Part model, mm, in its own coordinate system. Round coordinates to 2 decimals unless told otherwise and drop trailing zeros. Write each loop counter-clockwise with the first axis right and the second up, starting at its lowest first coordinate (ties: lowest second). Pieces come first, ordered by that corner, then holes. Notation, with made-up numbers: M 89.25,46 L 103.25,46 A16 cw 103.25,53 Z; hole C 3,33 d7. An arc over 180 degrees is marked long. One line per question, with ' | ' between items. Start each with the question number.
1) Saw through at A-A (z = 0). List the corners of the cut face in (x, y).
2) Saw through at B-B (y = 11.75). List the corners of the cut face in (x, z).
3) Saw through at C-C (x = 31.5). List the corners of the cut face in (y, z).
4) Wall check: probe 1 along Z at (x, y) = (18, 0); probe 2 along X at (y, z) = (12.5, 0.05); probe 3 along Y at (x, z) = (27, 0.15). Give the ranges that are in metal, low to high. Write a range as [from, to].
Autodesk Fusion 360 part; units mm, degrees
sketch "Sketch1" plane through (0, 0, 0) normal (1, 0, 0) x (0, 1, 0)
  circle A0 centre (0, 0) radius 1.3
  circle A1 centre (0, 0) radius 1.1476
  dimension "d1" = 2.6
  dimension "d2" = 2.2952
extrude "Extrude1" add sketch "Sketch1" along normal blind 20
equation "d2 = d1 - 0.012 in"

Autodesk Fusion 360 part; units mm, degrees
sketch "Sketch1" plane through (0, 0, 0) normal (1, 0, 0) x (0, 1, 0)
  circle A0 centre (0, 0) radius 1.3
  circle A1 centre (0, 0) radius 1.1476
  dimension "d1" = 2.6
  dimension "d2" = 2.2952
extrude "Extrude1" add sketch "Sketch1" along normal blind 7
equation "d2 = d1 - 0.012 in"

Autodesk Fusion 360 part; units mm, degrees
sketch "Sketch1" plane through (0, 0, 0) normal (1, 0, 0) x (0, 1, 0)
  circle A0 centre (0, 0) radius 1.3
  circle A1 centre (0, 0) radius 1.1476
  dimension "d1" = 2.6
  dimension "d2" = 2.2952
sketch "Sketch2" plane through (0, 0, 0) normal (0, 0, 1) x (1, 0, 0)
  line L0 (0, 0) -> (40.8, 0)
  line L1 (50.8, 10) -> (50.8, 25)
  arc A0 (40.8, 0) -> (50.8, 10) centre (40.8, 10) ccw
  point P0 (50.8, 0)
  dimension "d3" = 50.8
  dimension "d4" = 25
  dimension "d5" = 10
sweep "Sweep1" add profiles "Sketch1" path "Sketch2" along L0 A0 L1 section 1
equation "d2 = d1 - 0.012 in"
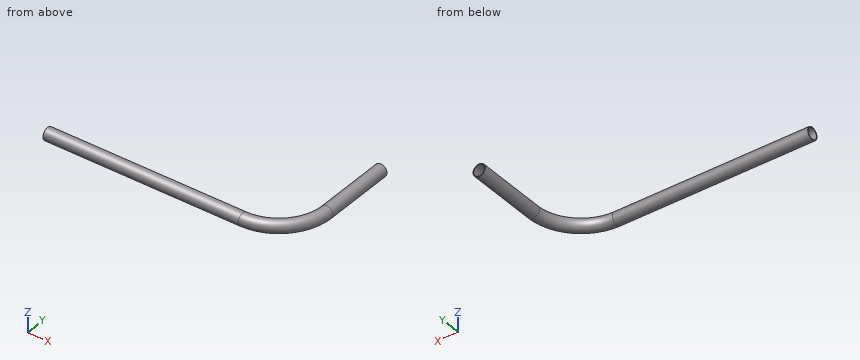
Answer key:
1) outline: M 0,-1.3 L 40.8,-1.3 A11.3 ccw 52.1,10 L 52.1,25 L 51.95,25 L 51.95,10 A11.15 cw 40.8,-1.15 L 0,-1.15 Z; M 0,1.15 L 40.8,1.15 A8.85 ccw 49.65,10 L 49.65,25 L 49.5,25 L 49.5,10 A8.7 cw 40.8,1.3 L 0,1.3 Z
2) outline: C 50.8,0 d2.6; hole C 50.8,0 d2.3
3) outline: C 0,0 d2.6; hole C 0,0 d2.3
4) probe 1: z = [-1.3, -1.15], [1.15, 1.3] | probe 2: x = [49.5, 49.65], [51.95, 52.1] | probe 3: y = [-1.29, -1.14], [1.14, 1.29]
